Verification items for the finished model (mm, model axes). Give positions to 0.01 mm unless a question says otherwise; leave off trailing zeros. Write each loop counter-clockwise with the first axis right and the second up, starting at its lowest first coordinate (ties: lowest second). Pieces come first, ordered by that corner, then holes.
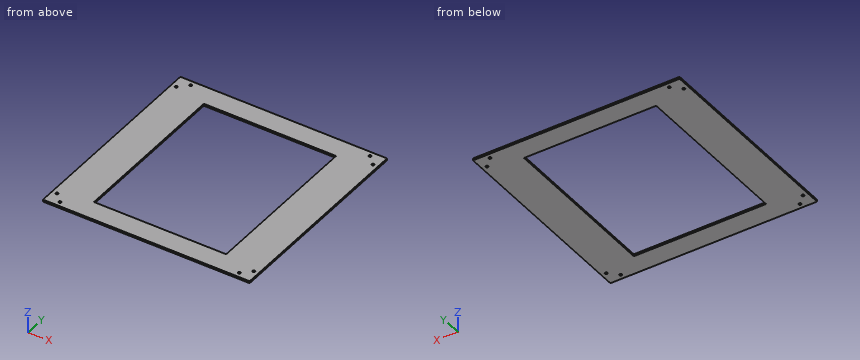
Autodesk Inventor part; units mm, degrees
ref_plane "YZ Plane" through (0, 0, 0) normal (1, 0, 0) x (0, 1, 0)
ref_plane "XZ Plane" through (0, 0, 0) normal (0, 1, 0) x (-1, 0, 0)
ref_plane "XY Plane" through (0, 0, 0) normal (0, 0, 1) x (1, 0, 0)
sketch "Skizze1" plane through (0, 0, 0) normal (0, 0, 1) x (1, 0, 0)
  line L0 (-250, -250) -> (250, -250)
  line L1 (250, -250) -> (250, 250)
  line L2 (250, 250) -> (-250, 250)
  line L3 (-250, 250) -> (-250, -250)
  line L4 (-250, -250) -> (250, 250) construction
  line L5 (250, -250) -> (-250, 250) construction
  point P0 (0, 0)
  dimension "d0" = 500
  dimension "d1" = 500
extrude "Extrusion1" add sketch "Skizze1" along normal blind 5
sketch "Skizze2" plane through (0, 0, 5) normal (0, 0, 1) x (1, 0, 0)
  line L0 (250, 250) -> (-250, 250)
  line L1 (-250, 250) -> (-250, -250)
  line L2 (0, -350) -> (0, 350)
  line L3 (-350, 0) -> (350, 0)
  point P0 (0, 0)
  point P1 (-238, 217)
  point P2 (-217, 238)
  point P3 (238, 217)
  point P4 (217, 238)
  point P5 (-238, -217)
  point P6 (-217, -238)
  point P7 (217, -238)
  point P8 (238, -217)
  dimension "d4" = 33
  dimension "d5" = 33
  dimension "d6" = 12
  dimension "d7" = 12
hole "Bohrung1" at (-238, 217, 5) at (-217, 238, 5) at (217, 238, 5) at (238, 217, 5) at (-238, -217, 5) at (-217, -238, 5) at (217, -238, 5) at (238, -217, 5) direction (0, 0, -1) diameter 6.1 end through all
sketch "Skizze3" plane through (0, 0, 5) normal (0, 0, 1) x (1, 0, 0)
  line L0 (-160, -200) -> (160, -200)
  line L1 (160, -200) -> (160, 200)
  line L2 (160, 200) -> (-160, 200)
  line L3 (-160, 200) -> (-160, -200)
  line L4 (-160, -200) -> (160, 200) construction
  line L5 (160, -200) -> (-160, 200) construction
  point P0 (0, 0)
  dimension "d15" = 320
  dimension "d16" = 400
extrude "Extrusion2" cut sketch "Skizze3" against normal through all
properties part number "Hinterwand"
Item 1: Sectioned sample at A-A on x = -76.5. Record the cut outline in (y, z), then the cut area to 3 significant figures.
Answer key:
outline: (-250, 0) - (-200, 0) - (-200, 5) - (-250, 5) - close; (200, 0) - (250, 0) - (250, 5) - (200, 5) - close
area: 500 mm2
Item 2: Sectioned sample at C-C on z = 3.7. State how many separate pieces and enclosed holes the cut face has, then the cut area to 3 significant figures.
Answer key:
separate pieces: 1
enclosed holes: 9
area: 122,000 mm2
Item 3: Scan lines: line 1 along Y through (x, z) = (238, 1.25); line 2 along Y through (x, z) = (217, 3.75). Record each from-to range of solid material in increasing order.
Answer key:
line 1: y = -250 to -220.05, -213.95 to 213.95, 220.05 to 250
line 2: y = -250 to -241.05, -234.95 to 234.95, 241.05 to 250
Item 4: Sectioned sample at B-B on y = 193. Record the cut outline in (x, z), then the cut area to 3 significant figures.
Answer key:
outline: (-250, 0) - (-160, 0) - (-160, 5) - (-250, 5) - close; (160, 0) - (250, 0) - (250, 5) - (160, 5) - close
area: 900 mm2
